from build123d import *

# Parameters (mm, degrees)
SKETCH_1_W      = 40
SKETCH_1_H      = 40
SKETCH_1_W_2    = 16
SKETCH_1_H_2    = 16
EXTRUDE_2_DEPTH = 15
SKETCH_2_W      = 16
SKETCH_2_H      = 16
EXTRUDE_3_DEPTH = 55


with BuildPart() as part:
    # 草图1 → 凸台-拉伸2 (new body)
    with BuildSketch(Plane.XY):
        Rectangle(SKETCH_1_W, SKETCH_1_H)
        Rectangle(SKETCH_1_W_2, SKETCH_1_H_2, mode=Mode.SUBTRACT)
    extrude(amount=EXTRUDE_2_DEPTH)

    # 草图2 → 凸台-拉伸3 (add)
    with BuildSketch(Plane.XY.offset(15)):
        Rectangle(SKETCH_2_W, SKETCH_2_H)
    extrude(amount=-EXTRUDE_3_DEPTH)


solid = part.part
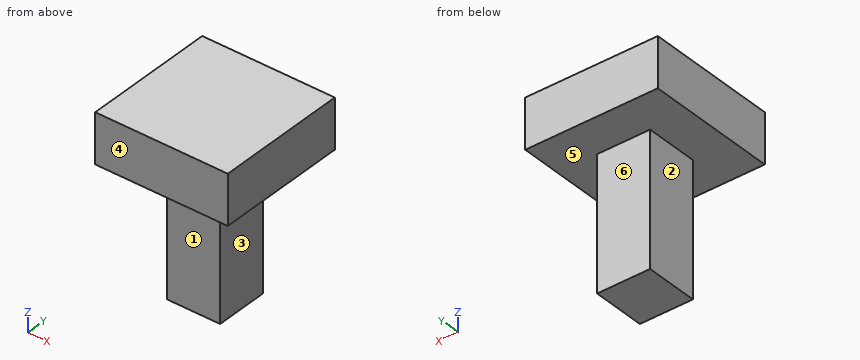
Read the model definition and answer for the solid it produces. Units are mm, in the model's axes. Face numbers are marked on the shaded views. A direction names the side the tool comes from. Coordinates: 2 decimals unless noted, no trailing zeros. Loops run counter-clockwise (first coordinate to the right, second up) from the corner with the lowest first, then second, coordinate; pieces in that order, holes last.
Q1. Each of these flat-tipped pins is pushed along its axis until it touches: pin 1 Ø5 at (x, z) = (1, -25) entering from -Y; pin 2 Ø13 at (y, z) = (3, -24) entering from -X; pin 3 Ø5 at (x, z) = (3.5, -19) entering from +Y. Where does it stop, or does it pass through?
Q2. Consider probe 1 along X at (y, z) = (5.5, -19.5); probe 2 along Z at (x, y) = (16, -9.5). Determine where each line is inside the solid, lowest interval first.
Q3. The part is cut by section C-C on z = -4.5. Write down the section's boundary in (x, y), and give its area (3 significant figures).
Q4. The part is cut by section A-A on y = -4. Write down the section's boundary in (x, z), and give its area (3 significant figures).
Q5. The mould has two halves that part along Y. Classify the marked faces 4, 5 and 6: +Y half, -Y half, draft (parallel to the pull), parting line (faces both ways), or undercut.
Q6. Which of the six approach directions +Z, -Z, +X, -X, +Y, -Y give full straight-line access (tool end or side, diameter ignored) to the marked faces 1, 2 and 3?
Q7. The part is cut by section D-D on x = -11. Write down the section's boundary in (y, z).
Results below:
1. pin 1: stops at y = -8
1. pin 2: stops at x = -8
1. pin 3: stops at y = 8
2. probe 1: x = -8 to 8
2. probe 2: z = 0 to 15
3. outline: (-8, -8) - (8, -8) - (8, 8) - (-8, 8) - close
3. area: 256 mm2
4. outline: (-20, 0) - (-8, 0) - (-8, -40) - (8, -40) - (8, 0) - (20, 0) - (20, 15) - (-20, 15) - close
4. area: 1,240 mm2
5. face 4: -Y half
5. face 5: draft
5. face 6: +Y half
6. face 1: -Z, +X, -X, -Y
6. face 2: -Z, -X, +Y, -Y
6. face 3: -Z, +X, +Y, -Y
7. outline: (-20, 0) - (20, 0) - (20, 15) - (-20, 15) - close
